from build123d import *

# Parameters (mm, degrees)
BOSS_EXTRUDE1_DEPTH                 = 6
FILLET1_R                           = 15
BOSS_EXTRUDE2_DEPTH                 = 30
F_16_0_16_DIAMETER_HOLE1_D          = 16
SKETCH4_W                           = 14
SKETCH4_H                           = 27
CUT_EXTRUDE1_DEPTH                  = 50
SKETCH5_W                           = 8
SKETCH5_H                           = 6.001
F_16_0_16_DIAMETER_HOLE2_AT_2_COUNT = 2
F_16_0_16_DIAMETER_HOLE2_AT_2_PITCH = 52.737557774
F_16_0_16_DIAMETER_HOLE2_AT_3_COUNT = 2
F_16_0_16_DIAMETER_HOLE2_AT_3_PITCH = 52.737557774


with BuildPart() as part:
    # Sketch1 → Boss-Extrude1 (new body)
    with BuildSketch(Plane(origin=(0, 0, 0), x_dir=(1, 0, 0), z_dir=(0, 1, 0))):
        Polygon((57.5, 0), (57.5, -45), (27.5, -45), (27.5, 0), (0, 0), (0, 30), (85, 30), (85, 0), align=None)
    extrude(amount=BOSS_EXTRUDE1_DEPTH)

    # Fillet1
    fillet1_edges = [part.edges().sort_by_distance(p)[0] for p in [
        (85, 3, -30),
        (85, 3, 0),
        (0, 3, -30),
        (0, 3, 0),
        (27.5, 3, 45),
        (57.5, 3, 45),
    ]]
    fillet(fillet1_edges, radius=FILLET1_R - 0.0001)  # a hair under: the kernel refuses the full size

    # Sketch2 → Boss-Extrude2 (add)
    with BuildSketch(Plane(origin=(57.5, 0, 0), x_dir=(0, 0, -1), z_dir=(1, 0, 0))):
        with BuildLine():
            Line((-17, 6), (30, 6))
            Line((30, 6), (30, 30))
            ThreePointArc((30, 30), (19.021918108, 44.450749971), (2.156776702, 37.749297731))
            Line((2.156776702, 37.749297731), (-17, 6))
        make_face()
    extrude(amount=-BOSS_EXTRUDE2_DEPTH)

    # Ø16.0 (16) Diameter Hole1 (through all)
    with Locations(Plane(origin=(57.5, 30, -15), x_dir=(0, 0, 1), z_dir=(1, 0, 0))):
        with Locations((0, 0)):
            Hole(F_16_0_16_DIAMETER_HOLE1_D / 2)

    # Sketch4 → Cut-Extrude1 (cut)
    with BuildSketch(Plane(origin=(0, 0, -30), x_dir=(-1, 0, 0), z_dir=(0, 0, -1))):
        with Locations((-42.5, 31.5)):
            Rectangle(SKETCH4_W, SKETCH4_H)
    extrude(amount=-CUT_EXTRUDE1_DEPTH, mode=Mode.SUBTRACT)

    # Sketch5 → Ø16.0 (16) Diameter Hole2 (revolve, cut)
    with BuildSketch(Plane(origin=(42.5, 0, 30), x_dir=(0, 0, -1), z_dir=(1, 0, 0))):
        with Locations((4, 3.0005)):
            Rectangle(SKETCH5_W, SKETCH5_H)
    f_16_0_16_diameter_hole2 = revolve(axis=Axis((42.5, -6.35, 30), (0, 1, 0)), mode=Mode.SUBTRACT)

    # Ø16.0 (16) Diameter Hole2 at 2: Ø16.0 (16) Diameter Hole2 ×2
    with Locations(*[Vector(-0.521450009453975, 0, -0.853281833651959) * (i * F_16_0_16_DIAMETER_HOLE2_AT_2_PITCH) for i in range(1, F_16_0_16_DIAMETER_HOLE2_AT_2_COUNT)]):
        add(f_16_0_16_diameter_hole2, mode=Mode.SUBTRACT)

    # Ø16.0 (16) Diameter Hole2 at 3: Ø16.0 (16) Diameter Hole2 ×2
    with Locations(*[Vector(0.5214500094539749, 0, -0.8532818336519591) * (i * F_16_0_16_DIAMETER_HOLE2_AT_3_PITCH) for i in range(1, F_16_0_16_DIAMETER_HOLE2_AT_3_COUNT)]):
        add(f_16_0_16_diameter_hole2, mode=Mode.SUBTRACT)


solid = part.part
CAD build for the part. Positions are in the model's coordinates, mm. A direction names the side the tool comes from. Coordinates: 2 decimals unless noted, no trailing zeros. Write each loop counter-clockwise with the first axis right and the second up, starting at its lowest first coordinate (ties: lowest second). Pieces come first, ordered by that corner, then holes. Notation, with made-up numbers: M 25.25,88.5 L 59.25,88.5 A15 cw 59.25,108.5 Z; hole C -3.75,79.5 d10. An arc over 180 degrees is marked long. Answer as a JSON object with one key per item and string values. Group by question number.
1) Pin check, flat tips, straight feed: pin 1 Ø21.5 at (y, z) = (28.5, -9.5) entering from -X; pin 2 Ø6.5 at (x, y) = (61.5, 4) entering from +Z; pin 3 Ø18.5 at (y, z) = (30, -15) entering from +X; pin 4 Ø12 at (y, z) = (12.5, 29) entering from -X. Stop position of each tip, or through.
2) Tool access for faces 4 (the face through (53.22, 3.04, 40.49)), 5 (the face through (74.5, 6, -21.9)), 6 (the face through (43, 18, -10)), 7 (the face through (20.1, 6, -8.5)), 8 (the face through (43, 6, 21)): list every direction of +Z, -Z, +X, -X, +Y, -Y with a clear straight run to the whole face (end or side of a thin tool).
3) Saw through at B-B (y = 32). Write the cut outline in (x, z).
4) Saw through at D-D (x = 52.5). Write the cut outline in (y, z).
5) Saw through at A-A (x = 68). Write the cut outline in (y, z).
6) Mould opens along X. For faces 1 (the face through (35.5, 28, -6)), 2 (the face through (80.49, 3.04, -25.72)), 3 (the face through (42.71, 15.041, 11.545)) say: +X half, -X half, draft (parallel to the pull), parting line (faces both ways), or undercut.
7) Saw through at C-C (z = 33). Write the cut outline in (x, y).
8) Wall check: line 1 (X direction, y = 2.25, z = -15); line 2 (X direction, y = 20.5, z = 3.5); line 3 (Y direction, x = 55.25, z = -15). Give the ranges that are in metal, low to high. Write a range as from..to.
Values follow:
{
 "1": {"pin 1": "stops at x = 27.5", "pin 2": "stops at z = 0", "pin 3": "stops at x = 57.5", "pin 4": "passes through"},
 "2": {"face 4": "+Z, +X, +Y, -Y", "face 5": "+Z, -Z, +X, +Y", "face 6": "+Z, -Z, +Y", "face 7": "+Z, -Z, -X, +Y", "face 8": "+Z, +X, -X, +Y"},
 "3": {"outline": "M 27.5,-29.87 L 35.5,-29.87 L 35.5,-22.75 L 27.5,-22.75 Z; M 27.5,-7.25 L 35.5,-7.25 L 35.5,1.31 L 27.5,1.31 Z; M 49.5,-29.87 L 57.5,-29.87 L 57.5,-22.75 L 49.5,-22.75 Z; M 49.5,-7.25 L 57.5,-7.25 L 57.5,1.31 L 49.5,1.31 Z"},
 "4": {"outline": "M 0,-30 L 30,-30 A15 ccw 37.75,-2.16 L 6,17 L 6,41.18 L 0,41.18 Z; hole C 30,-15 d16"},
 "5": {"outline": "M 0,-30 L 6,-30 L 6,-22.75 L 0,-22.75 Z; M 0,-7.25 L 6,-7.25 L 6,0 L 0,0 Z"},
 "6": {"face 1": "undercut", "face 2": "+X half", "face 3": "draft"},
 "7": {"outline": "M 27.8,0 L 35.08,0 L 35.08,6 L 27.8,6 Z; M 49.92,0 L 57.2,0 L 57.2,6 L 49.92,6 Z"},
 "8": {"line 1": "x = 0..7, 23..62, 78..85", "line 2": "x = 27.5..35.5, 49.5..57.5", "line 3": "y = 0..22, 38..45"}
}
